Input: part model. Units: mm. Frame: model coordinates. Face numbers are marked on the shaded views. A direction names the side the tool comes from. Coordinates: 2 decimals unless noted, no trailing zeros. Order: outer loops, then holes, each group sorted by start corner. A loop starts at its lowest first (then second) coordinate and runs counter-clockwise, first axis right, second up. Notation, with made-up numbers: (9, 76.5) - (42, 76.5) arc R14 ccw to (42, 83.5) - close; hole circle Ø9 at (29, -24.75). An arc over 180 degrees is marked (long way). Use a Markdown table: item, result. Add a question column.
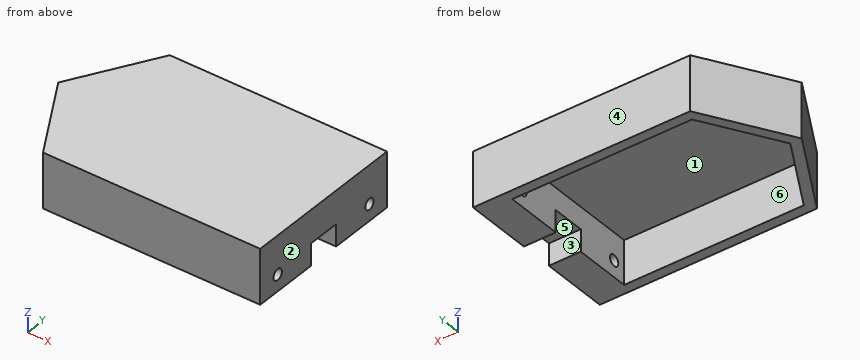
Autodesk Inventor part; units mm, degrees
ref_plane "YZ Plane" through (0, 0, 0) normal (1, 0, 0) x (0, 1, 0)
ref_plane "XZ Plane" through (0, 0, 0) normal (0, 1, 0) x (-1, 0, 0)
ref_plane "XY Plane" through (0, 0, 0) normal (0, 0, 1) x (1, 0, 0)
sketch "Sketch1" plane through (0, 0, 0) normal (0, 0, 1) x (1, 0, 0)
  line L0 (44.453, 0) -> (22.2265, -38.4974)
  line L1 (22.2265, -38.4974) -> (-22.2265, -38.4974)
  line L2 (-22.2265, -38.4974) -> (-44.453, 0)
  line L3 (-44.453, 0) -> (-22.2265, 38.4974)
  line L4 (-22.2265, 38.4974) -> (22.2265, 38.4974)
  line L5 (22.2265, 38.4974) -> (44.453, 0)
  line L6 (22.2265, 38.4974) -> (77.5, 38.4974)
  line L7 (22.2265, -38.4974) -> (77.5, -38.4974)
  line L8 (77.5, -38.4974) -> (77.5, 38.4974)
  point P0 (0, 0)
  point P1 (0, 0)
  dimension "d1" = 99.7265
  dimension "d2" = 76.9948
extrude "Extrusion1" add sketch "Sketch1" along normal blind 15
sketch "Sketch2" plane through (77.5, -38.4974, 0) normal (1, 0, 0) x (0, 0, -1)
  circle A0 centre (-7.5, 65.9974) radius 2.5
  circle A1 centre (-7.5, 10.9974) radius 2.5
  line L0 (-7.5, 65.9974) -> (-7.5, 10.9974) construction
  line L1 (0, 0) -> (0, 76.9948) construction
  line L2 (0, 76.9948) -> (-15, 76.9948) construction
  point P0 (0, 38.4974)
  point P1 (-7.5, 38.4974)
  point P2 (0, 38.4974)
  point P3 (-7.5, 76.9948)
  dimension "d5" = 5
  dimension "d6" = 5
  dimension "d7" = 55
extrude "Extrusion2" cut sketch "Sketch2" against normal blind 25
sketch "Sketch3" plane through (0, 0, 0) normal (0, 0, -1) x (-1, 0, 0)
  line L0 (-77.5, -38.4974) -> (-77.5, 38.4974)
  line L1 (-77.5, 7.5) -> (-62.5, 7.5)
  line L2 (-62.5, 7.5) -> (-62.5, -7.5)
  line L3 (-62.5, -7.5) -> (-77.5, -7.5)
  line L4 (-77.5, -7.5) -> (-77.5, 7.5)
  line L5 (-77.5, 38.4974) -> (22.2265, 38.4974)
  line L6 (22.2265, 38.4974) -> (44.453, 0)
  line L7 (44.453, 0) -> (22.2265, -38.4974)
  line L8 (22.2265, -38.4974) -> (-77.5, -38.4974)
  line L9 (38.6795, 0) -> (19.3397, 33.4974)
  line L10 (19.3397, 33.4974) -> (-72.5, 33.4974)
  line L11 (-72.5, 33.4974) -> (-72.5, -33.4974) construction
  line L12 (-72.5, -33.4974) -> (19.3397, -33.4974)
  line L13 (19.3397, -33.4974) -> (38.6795, 0)
  line L14 (-62.5, 7.5) -> (-62.5, 33.4974)
  line L15 (-62.5, -7.5) -> (-62.5, -33.4974)
  line L16 (19.3397, 33.4974) -> (-62.5, 33.4974)
  line L17 (-62.5, -33.4974) -> (19.3397, -33.4974)
  point P0 (0, 0)
  point P1 (-77.5, 0)
  dimension "d10" = 15
  dimension "d11" = 15
  dimension "d12" = 5
extrude "Extrusion3" cut sketch "Sketch3" against normal blind 10 contours L0 L1 L2 L3 | L2 L14 L10 L9 L13 L12 L15
sketch "Sketch5" plane through (0, 0, 15) normal (0, 0, 1) x (1, 0, 0)
  line L0 (77.5, 38.4974) -> (-22.2265, 38.4974)
  line L1 (-22.2265, 38.4974) -> (-44.453, 0)
  line L2 (-44.453, 0) -> (-22.2265, -38.4974)
  line L3 (-22.2265, -38.4974) -> (77.5, -38.4974)
  line L4 (77.5, -38.4974) -> (77.5, 38.4974)
  line L5 (77, -37.9974) -> (-21.9378, -37.9974)
  line L6 (-21.9378, -37.9974) -> (-43.8756, 0)
  line L7 (-43.8756, 0) -> (-21.9378, 37.9974)
  line L8 (-21.9378, 37.9974) -> (77, 37.9974)
  line L9 (77, 37.9974) -> (77, -37.9974)
  point P0 (0, 0)
  dimension "d15" = 0.5
extrude "Extrusion4" cut sketch "Sketch5" against normal through all
sketch "Sketch6" plane through (0, 0, 15) normal (0, 0, 1) x (1, 0, 0)
  line L0 (77, -37.9974) -> (77, 37.9974)
  line L1 (77, 37.9974) -> (-21.9378, 37.9974)
  line L2 (-21.9378, 37.9974) -> (-43.8756, 0)
  line L3 (-43.8756, 0) -> (-21.9378, -37.9974)
  line L4 (-21.9378, -37.9974) -> (77, -37.9974)
  point P0 (0, 0)
extrude "Extrusion5" add sketch "Sketch6" along normal blind 10
sketch "Sketch7" plane through (0, 0, 10) normal (0, 0, -1) x (-1, 0, 0)
  line L0 (-77, 7.5) -> (-77, -7.5)
  line L1 (-62.5, -7.5) -> (-77, -7.5)
  line L2 (-62.5, -27.5) -> (-62.5, -7.5)
  line L3 (-62.5, -33.4974) -> (-62.5, -27.5)
  line L4 (19.3397, -33.4974) -> (-62.5, -33.4974)
  line L5 (38.6795, 0) -> (19.3397, -33.4974)
  line L6 (19.3397, 33.4974) -> (38.6795, 0)
  line L7 (-62.5, 33.4974) -> (19.3397, 33.4974)
  line L8 (-62.5, 27.5) -> (-62.5, 33.4974)
  line L9 (-62.5, 7.5) -> (-62.5, 27.5)
  line L10 (-77, 7.5) -> (-62.5, 7.5)
  line L11 (-62.5, 7.5) -> (-62.5, -7.5)
  point P0 (0, 0)
extrude "Extrusion6" cut sketch "Sketch7" against normal blind 10 contours L9 L8 L7 L6 L5 L4 L3 L2 L11
properties part number "TARM06" material "ABS Plastic"
1) Cut plane A-A (z = 7.5). Return the cut outline in (x, y).
2) Cut plane D-D (y = -6). Return the cut outline in (x, z).
3) Cut plane B-B (y = 27.5). Return the cut outline in (x, z), and give its area (3 significant figures).
4) Reachability of the marked faces 4, 5 and 6 from +Z, -Z, +X, -X, +Y, -Y: full face, straight path, thin tool, end or side. Return the list, or none.
5) Contact query for flat-ended pins moving along their axis: P1, Ø7, axis at x = 72, y = 1.5, coming from the -Z side; P2, Ø5, axis at x = 7, y = -22, coming from the -Z side; P3, Ø4, axis at y = -27.5, z = 7.5, coming from the -X side. Output: stop coordinate, or through.
6) Pull-direction query (X, two-part tool) for the marked faces 1, 2 and 3; classes: pulls with the +X half, pulls with the -X half, needs draft (parallel to the pull), parting line crosses it, or undercut.
7) Cut plane C-C (x = 13.5). Return the cut outline in (y, z).
8) Material intervals for L1, parallel to Y at x = 65.5, z = 7.5; L2, parallel to Z at x = 66.25, y = 27.5; L3, parallel to Y at x = -7, z = 9.5, sorted ascending.
Computed:
| question | item | result |
|---|---|---|
| 1 | outline | (-43.88, 0) - (-21.94, -38) - (77, -38) - (77, -30) - (62.5, -30) - (62.5, -33.5) - (-19.34, -33.5) - (-38.68, 0) - (-19.34, 33.5) - (62.5, 33.5) - (62.5, 30) - (77, 30) - (77, 38) - (-21.94, 38) - close; (62.5, -25) - (77, -25) - (77, -7.5) - (62.5, -7.5) - close; (62.5, 7.5) - (77, 7.5) - (77, 25) - (62.5, 25) - close |
| 2 | outline | (-40.41, 0) - (-35.22, 0) - (-35.22, 20) - (62.5, 20) - (62.5, 10) - (77, 10) - (77, 25) - (-40.41, 25) - close |
| 3 | outline | (-28, 0) - (-22.8, 0) - (-22.8, 20) - (62.5, 20) - (62.5, 10) - (77, 10) - (77, 25) - (-28, 25) - close; (62.5, 0) - (77, 0) - (77, 5) - (62.5, 5) - close |
| 3 | area | 846 mm2 |
| 4 | face 4 | +Z, -Z, +X, -X, +Y |
| 4 | face 5 | -Z, +X |
| 4 | face 6 | -Z |
| 5 | P1 | stops at z = 10 |
| 5 | P2 | stops at z = 20 |
| 5 | P3 | stops at x = -29.15 |
| 6 | face 1 | undercut |
| 6 | face 2 | pulls with the +X half |
| 6 | face 3 | needs draft |
| 7 | outline | (-38, 0) - (-33.5, 0) - (-33.5, 20) - (33.5, 20) - (33.5, 0) - (38, 0) - (38, 25) - (-38, 25) - close |
| 8 | L1 | y = -38 to -30, -25 to -7.5, 7.5 to 25, 30 to 38 |
| 8 | L2 | z = 0 to 5, 10 to 25 |
| 8 | L3 | y = -38 to -33.5, 33.5 to 38 |
